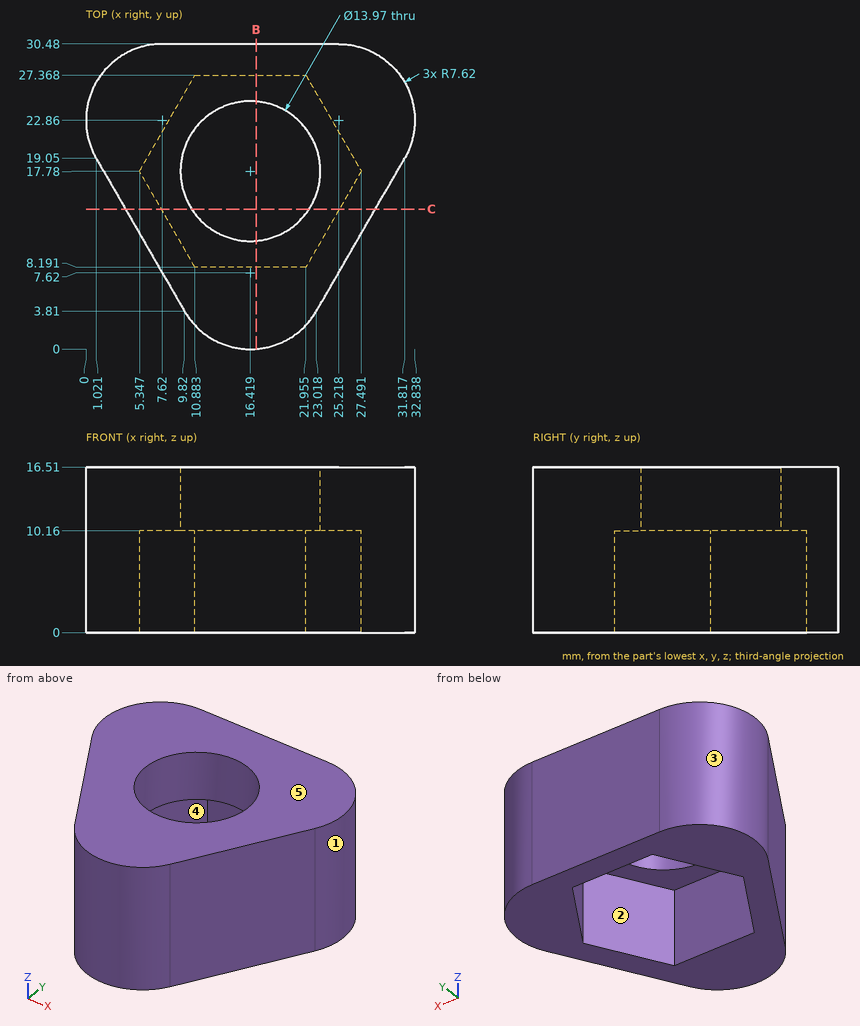
Print and shaded views of the part. All mm, measured from the part's lowest x, y and z. A direction names the side the tool comes from. Coordinates: 2 decimals unless noted, no trailing zeros. Loops run counter-clockwise (first coordinate to the right, second up) from the corner with the lowest first, then second, coordinate; pieces in that order, holes last. Notation, with made-up numbers: (-9.75, 85) -> (45.25, 85) arc R18 ccw to (45.25, 120) -> close; hole circle Ø1 at (54.25, 28.5). An arc over 180 degrees is marked (long way). Use one line per item in the form item = value. Start each with the question number.
(1) Tool access for the marked faces 4 and 5: list every direction of +Z, -Z, +X, -X, +Y, -Y with a clear straight run to the whole face (end or side of a thin tool).
(2) Flat gauge pins, fed straight in: pin 1 (6 mm diameter, centred on x = 21, z = 12.5, fed in from -Y); pin 2 (2 mm diameter, centred on y = 26.5, z = 2.5, fed in from +X) (1 decimal); pin 3 (18 mm diameter, centred on x = 16.42, y = 17.78, fed in from -Z). Where does each tip first touch, or does it go through?
(3) Probe probe 1 along X at (y, z) = (26, 5) (1 decimal); probe 2 along X at (y, z) = (25, 9.5) (1 decimal); probe 3 along Y at (x, z) = (12.5, 1.25) (1 decimal). List the from-to ranges inside material, lowest first. Write a range as from..to.
(4) Cut at B-B on x = 17. Give the cut face in (y, z), and give its area (3 significant figures).
(5) Pull direction X, two halves, no side cores. Call the marked faces 1, 2 and 3: pulls with the +X half, pulls with the -X half, needs draft (parallel to the pull), parting line crosses it, or undercut.
(6) Cut at C-C on y = 14. Give the cut face in (x, z) (1 decimal).
Values:
q1.face_4 = -Z
q1.face_5 = +Z, +X, -X, +Y, -Y
q2.pin_1 = 0.17
q2.pin_2 = 32.4
q2.pin_3 = 10.16
q3.probe_1 = 0.7..10.1, 22.7..32.2
q3.probe_2 = 0.3..9.5, 23.3..32.5
q3.probe_3 = 1.1..8.2, 27.4..30.5
q4.outline = (0.02, 0) -> (8.19, 0) -> (8.19, 10.16) -> (10.82, 10.16) -> (10.82, 16.51) -> (0.02, 16.51) -> close; (24.74, 10.16) -> (27.37, 10.16) -> (27.37, 0) -> (30.48, 0) -> (30.48, 16.51) -> (24.74, 16.51) -> close
q4.area = 220 mm2
q5.face_1 = pulls with the +X half
q5.face_2 = undercut
q5.face_3 = pulls with the -X half
q6.outline = (3.9, 0) -> (7.5, 0) -> (7.5, 10.2) -> (10.5, 10.2) -> (10.5, 16.5) -> (3.9, 16.5) -> close; (22.3, 10.2) -> (25.3, 10.2) -> (25.3, 0) -> (28.9, 0) -> (28.9, 16.5) -> (22.3, 16.5) -> close
